Verification items for this drawing (mm, ordinates from the low corner). Coordinates: 2 decimals unless noted, no trailing zeros. Write each loop counter-clockwise with the first axis right and the second up, starting at its lowest first coordinate (ties: lowest second). Pieces come first, ordered by that corner, then holes. Notation, with made-up numbers: (49, 42.5) -> (105, 42.5) arc R9 cw to (105, 53.5) -> close; hole circle Ø9 at (41, 80.25). An arc over 180 degrees is marked (long way). Put each result on its own line as item: value. Start each with the question number.
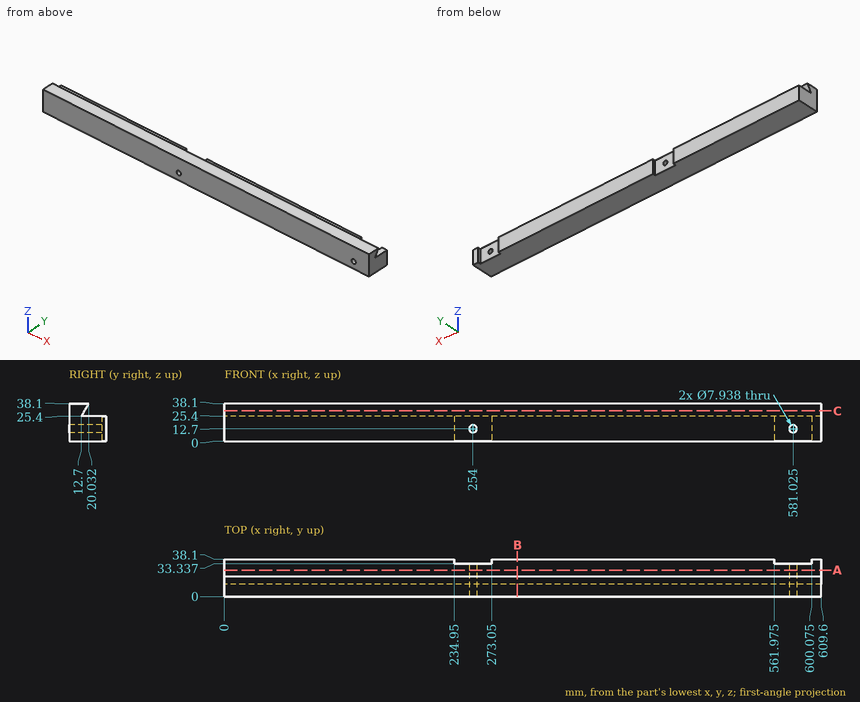
Item 1: Scan lines: line 1 along X through (y, z) = (17, 12); line 2 along X through (y, z) = (23.5, 11.5); line 3 along Z through (x, y) = (254, 19.5) (1 decimal). Record each from-to range of solid material in increasing order. Write a range as [from, to].
Item 2: Section check C-C, the plane z = 31. Enter the section's corners in (x, y), and give its area (3 significant figures).
Item 3: Go/stop test with flat-tipped pins: P1, Ø5, axis at x = 264.5, y = 26, coming from the +Z side; P2, Ø6.5, axis at x = 581.025, z = 12.7, coming from the +Y side; P3, Ø20.5, axis at x = 255.5, z = 9.5, coming from the +Y side. Record where each tip stops, or that it passes through.
Item 4: Section check B-B, the plane x = 299.5. Enter the section's corners in (y, z).
Item 5: Section check A-A, the plane y = 27. Enter the section's corners in (x, z) (1 decimal), and give its area (3 significant figures).
From the geometry:
1. line 1: [0, 250.09], [257.91, 577.12], [584.93, 609.6]
1. line 2: [0, 250.22], [257.78, 577.24], [584.81, 609.6]
1. line 3: [0, 8.7], [16.7, 25.4], [37.2, 38.1]
2. outline: (0, 0) -> (609.6, 0) -> (609.6, 15.93) -> (0, 15.93) -> close
2. area: 9,710 mm²
3. P1: z = 25.4
3. P2: through
3. P3: y = 33.34
4. outline: (0, 0) -> (38.1, 0) -> (38.1, 25.4) -> (12.7, 25.4) -> (20.03, 38.1) -> (0, 38.1) -> close
5. outline: (0, 0) -> (609.6, 0) -> (609.6, 25.4) -> (0, 25.4) -> close; hole circle Ø7.9 at (254, 12.7); hole circle Ø7.9 at (581, 12.7)
5. area: 15,400 mm²
